from build123d import *

# Parameters (mm, degrees)
F1_DEPTH = 5


with BuildPart() as f1:
    # F0 (on Top) → F1 (new body)
    with BuildSketch(Plane.XY):
        with BuildLine():
            Line((12.124356, 21), (24.248711, 0))
            Line((24.248711, 0), (33.486316, 16))
            Line((33.486316, 16), (30.599564, 21))
            Line((30.599564, 21), (28.599564, 21))
            ThreePointArc((28.599564, 21), (21.36196, 16.730604), (14.124356, 21))
            Line((14.124356, 21), (12.124356, 21))
        make_face()
        with BuildLine():
            Line((-9.814955, -17), (-19.629909, 0))
            Line((-19.629909, 0), (-9.814955, 17))
            Line((-9.814955, 17), (9.814955, 17))
            Line((9.814955, 17), (19.629909, 0))
            Line((19.629909, 0), (9.814955, -17))
            Line((9.814955, -17), (9.814955, -20.966555))
            ThreePointArc((9.814955, -20.966555), (11.983839, -20.1783), (13.567731, -18.5))
            Line((13.567731, -18.5), (24.248711, 0))
            Line((24.248711, 0), (12.124356, 21))
            Line((12.124356, 21), (-9.237604, 21))
            ThreePointArc((-9.237604, 21), (-11.737604, 20.330127), (-13.567731, 18.5))
            Line((-13.567731, 18.5), (-24.248711, 0))
            Line((-24.248711, 0), (-12.124356, -21))
            Line((-12.124356, -21), (-9.814955, -21))
            Line((-9.814955, -21), (-9.814955, -17))
        make_face()
        with BuildLine():
            Line((-14.124356, -21), (-12.124356, -21))
            Line((-12.124356, -21), (-24.248711, 0))
            Line((-24.248711, 0), (-33.486316, -16))
            Line((-33.486316, -16), (-30.599564, -21))
            Line((-30.599564, -21), (-28.599564, -21))
            ThreePointArc((-28.599564, -21), (-21.36196, -16.730604), (-14.124356, -21))
        make_face()
    extrude(amount=F1_DEPTH)


solid = f1.part
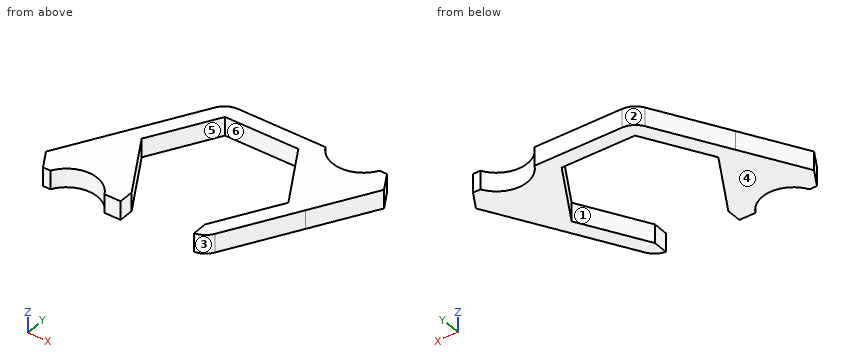
The model under review builds one solid part; all positions refer to its coordinate system, in mm. Face numbers are marked on the shaded views. A direction names the side the tool comes from. Coordinates: 2 decimals unless noted, no trailing zeros. Loops run counter-clockwise (first coordinate to the right, second up) from the corner with the lowest first, then second, coordinate; pieces in that order, holes last. Notation, with made-up numbers: M 80,-17 L 134,-17 A14 ccw 134,10 Z; hole C 40,50 d2. An arc over 180 degrees is marked long. Put each result on its own line as item: value. Start each with the question number.
Q1. For the marked faces 4, 5 and 6, list the 3-axis set-ups (+Z, -Z, +X, -X, +Y, -Y) from which the entire face can be reached by the end or side of a thin tool; tool diameter is ignored.
Q2. Add section B-B (z = 1.45). Write out the cut boundary in (x, y), and give its area (3 significant figures).
Q3. Wall thickness on line 1 (X direction, y = 0, z = 0.7); line 2 (X direction, y = -18, z = 2.45); line 3 (X direction, y = -7, z = 0.45): over which ranges is each line inside the solid? List them lowest first.
Q4. Add section A-A (y = 9.5). Write out the cut boundary in (x, z), and give its area (3 significant figures).
Q5. Add section D-D (x = -5). Write out the cut boundary in (y, z).
Q6. Clearance check with flat-ended pins moving along their axes: pin 1 (1.2 mm diameter, centred on y = -19.5, z = 2.5, fed in from +X); pin 2 (1 mm diameter, centred on y = 10, z = 3.5, fed in from -X); pin 3 (3 mm diameter, centred on x = -7, z = 2.5, fed in from -Y). State where each tip first meets the part, or that it passes through.
Q7. Add section C-C (y = -6). Write out the cut boundary in (x, z), and give its area (3 significant figures).
Q8. The part is to be moulded in two halves that separate along X. For the marked faces 1, 2 and 3, say which applies: +X half, -X half, draft (parallel to the pull), parting line (faces both ways), or undercut.
Answers:
1. face 4: -Z, +X, -X, +Y, -Y
1. face 5: +Z, -Z
1. face 6: +Z, -Z, -Y
2. outline: M -33.49,-16 L -30.6,-21 L -28.6,-21 A8.27 cw -14.12,-21 L -9.81,-21 L -9.81,-17 L -19.63,0 L -9.81,17 L 9.81,17 L 19.63,0 L 9.81,-17 L 9.81,-20.97 A5 ccw 13.57,-18.5 L 33.49,16 L 30.6,21 L 28.6,21 A8.27 cw 14.12,21 L -9.24,21 A5 ccw -13.57,18.5 Z
2. area: 838 mm^2
3. line 1: x = -24.25 to -19.63, 19.63 to 24.25
3. line 2: x = -32.33 to -25.76, -16.96 to -9.81, 9.81 to 13.86
3. line 3: x = -28.29 to -15.59, 15.59 to 20.21
4. outline: M -18.76,0 L -14.15,0 L -14.15,5 L -18.76,5 Z; M 14.15,0 L 29.73,0 L 29.73,5 L 14.15,5 Z
4. area: 101 mm^2
5. outline: M 17,0 L 21,0 L 21,5 L 17,5 Z
6. pin 1: stops at x = 13.31
6. pin 2: stops at x = -18.76
6. pin 3: stops at y = 17
7. outline: M -27.71,0 L -16.17,0 L -16.17,5 L -27.71,5 Z; M 16.17,0 L 20.78,0 L 20.78,5 L 16.17,5 Z
7. area: 80.8 mm^2
8. face 1: undercut
8. face 2: -X half
8. face 3: +X half
